For this review, take the finished solid that the model builds, in its own axes (mm). Round coordinates to 2 decimals unless told otherwise and drop trailing zeros. Order: outer loops, then holes, each group sorted by start corner. A loop starts at its lowest first (then second) coordinate and runs counter-clockwise, first axis right, second up. Notation, with made-up numbers: (-19, -27.75) -> (6, -27.75) arc R25 ccw to (6, -1.75) -> close; hole circle Ø3 at (-24, 54). An arc over 180 degrees is marked (long way). Use a Markdown table: item, result. Add a question column.
1) Wall thickness on line 1 along X through (y, z) = (15, -8.5); line 2 along Y through (x, z) = (41, -5.5); line 3 along Y through (x, z) = (78.5, -10): over which ranges is each line inside the solid? List them lowest first. Write a range as [from, to].
2) Consider section A-A (x = 56). State the section outline as (y, z) points.
3) Clearance check with flat-ended pins moving along their axes: P1, Ø4, axis at x = 26.5, z = -3.5, coming from the -Y side; P2, Ø10, axis at x = 67.5, z = -7.5, coming from the -Y side; P3, Ø5, axis at x = 58, z = 12.5, coming from the +Y side. State where each tip first meets the part, or that it passes through.
```python
from build123d import *


with BuildPart() as part:
    # Sketch1 → Revolve1 (revolve)
    with BuildSketch(Plane.XY, mode=Mode.PRIVATE) as revolve1_sk:
        Polygon((4, 16.5), (4, 17.5), (1.5, 17.5), (0, 16), (0, 0), (88, 0), (88, 16), (86.5, 17.5), (84, 17.5), (84, 16.5), (82, 16.5), (82, 17.5), (6, 17.5), (6, 16.5), align=None)
    revolve(revolve1_sk.sketch.rotate(Axis((-2, 0, 0), (1, 0, 0)), 90), axis=Axis((-2, 0, 0), (1, 0, 0)))


solid = part.part
```
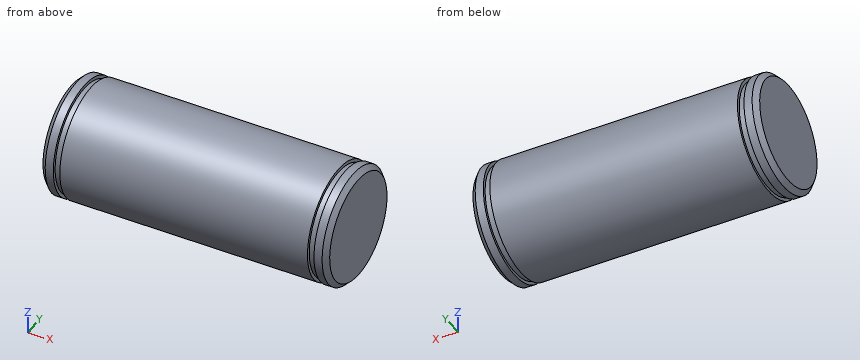
Results list:
| question | item | result |
|---|---|---|
| 1 | line 1 | [1.24, 4], [6, 82], [84, 86.76] |
| 1 | line 2 | [-16.61, 16.61] |
| 1 | line 3 | [-14.36, 14.36] |
| 2 | outline | circle Ø35 at (0, 0) |
| 3 | P1 | y = -17.44 |
| 3 | P2 | y = -17.32 |
| 3 | P3 | y = 14.36 |
